Here's how the part is built. I have some questions about the finished solid (model axes, mm). A direction names the side the tool comes from. Give positions to 0.01 mm unless a question says otherwise; leave off trailing zeros. Order: outer loops, then holes, each group sorted by start corner. A loop starts at its lowest first (then second) coordinate and runs counter-clockwise, first axis right, second up. Notation, with made-up numbers: M 34.5,-28 L 45.5,-28 A30 ccw 45.5,3 Z; hole C 22,-2 d5. An arc over 180 degrees is marked long. Use one line per item in the form item = value.
from build123d import *

# Parameters (mm, degrees)
F1_DEPTH  = 14
F2_R      = 3
F3_DEPTH  = 6.001
F4_R      = 1.75
F5_DEPTH  = 10.001
F7_DEPTH  = 6.0010001
F8_R      = 1.75
F9_DEPTH  = 6.001
F11_DEPTH = 10.0010001


with BuildPart() as f1:
    # F0 (on Top) → F1 (new body)
    with BuildSketch(Plane.XY):
        with BuildLine():
            Line((0.5, 11.7459666924), (0.5, 3.9686269666))
            ThreePointArc((0.5, 3.9686269666), (0, -4), (-0.5, 3.9686269666))
            Line((-0.5, 3.9686269666), (-0.5, 11.7459666924))
            Line((-0.5, 11.7459666924), (-2, 11.7459666924))
            Line((-2, 11.7459666924), (-2, 7.7459666924))
            ThreePointArc((-2, 7.7459666924), (-7.9996074848, -0.0792470114), (-1.8461538462, -7.7840680866))
            ThreePointArc((-1.8461538462, -7.7840680866), (0.9223227028, -9.5482422759), (2, -12.6491106407))
            Line((2, -12.6491106407), (2, -16))
            Line((2, -16), (8, -16))
            Line((8, -16), (8, 0))
            ThreePointArc((8, 0), (6.3245553203, 4.8989794856), (2, 7.7459666924))
            Line((2, 7.7459666924), (2, 11.7459666924))
            Line((2, 11.7459666924), (0.5, 11.7459666924))
        make_face()
    extrude(amount=F1_DEPTH)

    # F2 (on face) → F3 (cut, through all)
    with BuildSketch(Plane(origin=(-2, 0, 0), x_dir=(0, -1, 0), z_dir=(-1, 0, 0))):
        with Locations((-7.7459666924, 7)):
            Circle(F2_R)
    extrude(amount=F3_DEPTH, mode=Mode.SUBTRACT)

    # F4 (on face) → F5 (cut, through all)
    with BuildSketch(Plane(origin=(-2, 0, 0), x_dir=(0, -1, 0), z_dir=(-1, 0, 0))):
        with Locations((-7.7459666924, 7)):
            Circle(F4_R)
    extrude(amount=-F5_DEPTH, mode=Mode.SUBTRACT)

    # F6 (on face) → F7 (cut, through all)
    with BuildSketch(Plane.YZ.offset(2)):
        Polygon((3.7459666924, 4.6905989232), (7.7459666924, 2.3811978465), (11.7459666924, 4.6905989232), (11.7459666924, 9.3094010768), (7.7459666924, 11.6188021535), (3.7459666924, 9.3094010768), align=None)
    extrude(amount=F7_DEPTH, mode=Mode.SUBTRACT)

    # F8 (on face) → F9 (cut, through all)
    with BuildSketch(Plane(origin=(2, 0, 0), x_dir=(0, -1, 0), z_dir=(-1, 0, 0))):
        with Locations((12, 7)):
            Circle(F8_R)
    extrude(amount=-F9_DEPTH, mode=Mode.SUBTRACT)

    # F10 (on face) → F11 (cut, through all)
    with BuildSketch(Plane(origin=(2, 0, 0), x_dir=(0, -1, 0), z_dir=(-1, 0, 0))):
        Polygon((15.8407900553, 9.3094010768), (11.8407900553, 11.6188021535), (7.8407900553, 9.3094010768), (7.8407900553, 4.6905989232), (11.8407900553, 2.3811978465), (15.8407900553, 4.6905989232), align=None)
    extrude(amount=F11_DEPTH, mode=Mode.SUBTRACT)


solid = f1.part
Q1. On a 3-axis mill with a long thin cutter (end or side, diameter ignored), from which of +Z, -Z, +X, -X, +Y, -Y can I reach the whole of each face in a straight line? I mean faces 1 (the face through (0.5, 10, 7)), 2 (the face through (2, 9, 5)), 3 (the face through (8, -8, 7)), 4 (the face through (-2, 10, 7)), 5 (the face through (0, -7.841, 7)). Say none if no direction works.
Found:
face_1 = +Z, -Z, +Y
face_2 = +X, +Y
face_3 = +Z, -Z, +X, +Y, -Y
face_4 = -X, +Y
face_5 = -X, -Y
Q2. I want a section at D-D on x = 6.75. Write out the boundary of the cut face in (y, z), then the cut area to 3 significant figures.
Found:
outline = M -16,0 L 4.29,0 L 4.29,4.37 L 3.75,4.69 L 3.75,9.31 L 4.29,9.63 L 4.29,14 L -16,14 Z; hole C -12,7 d3.5
area = 272 mm²
Q3. I want a section at B-B on x = -1.25. Write out the boundary of the cut face in (y, z), then the cut area to 3 significant figures.
Found:
outline = M -7.97,0 L -3.8,0 L -3.8,14 L -7.97,14 L -7.97,9.38 L -7.84,9.31 L -7.84,4.69 L -7.97,4.62 Z; M 3.8,0 L 11.75,0 L 11.75,14 L 3.8,14 Z; hole C 7.75,7 d3.5
area = 159 mm²
Q4. Thinking about a two-plate mould opening in Z: for faces 6 (the face through (-0.5, 10, 7)), 7 (the face through (2, -5, 14)), 8 (the face through (-1.26, 9.135, 5.935)), which applies, +Z half, -Z half, draft (parallel to the pull), parting line (faces both ways), or undercut?
Found:
face_6 = draft
face_7 = +Z half
face_8 = undercut
Q5. I'm going to push flat-ended pins straight in: pin 1 Ø1.8 at (x, z) = (1, 7) entering from -Y; pin 2 Ø5.5 at (y, z) = (-12, 7) entering from -X; pin 3 Ø6.5 at (y, z) = (7.5, 7) entering from +X; pin 4 Ø6.5 at (x, y) = (0, 0) entering from -Z. Where does each tip first touch, or does it pass through?
Found:
pin_1 = -7.84
pin_2 = 2
pin_3 = 2
pin_4 = through
Q6. I want a section at C-C on y = 0.75. Write out the boundary of the cut face in (x, z), then the cut area to 3 significant figures.
Found:
outline = M -7.96,0 L -3.93,0 L -3.93,14 L -7.96,14 Z; M 3.93,0 L 7.96,0 L 7.96,14 L 3.93,14 Z
area = 113 mm²
Q7. I need wall thicknesses on L1, parallel to Y at x = 1, z = 7.75; L2, parallel to Y at x = 4.1, z = 7; L3, parallel to Y at x = -1, z = 7.25. Which ranges of each line are inside material? Lowest first, please.
Found:
L1 = -7.84 to -3.87, 3.87 to 6.16, 9.33 to 11.75
L2 = -16 to -13.75, -10.25 to 3.75
L3 = -7.84 to -3.87, 3.87 to 6.01, 9.48 to 11.75
Q8. I want a section at A-A on z = 7. Write out the boundary of the cut face in (x, y), then the cut area to 3 significant figures.
Found:
outline = M -6.44,4.75 A8 ccw -1.85,-7.78 A5 cw -1.63,-7.84 L 2,-7.84 L 2,-10.25 L 8,-10.25 L 8,0 A8 ccw 7.07,3.75 L 2,3.75 L 2,6 L 0.5,6 L 0.5,3.97 A4 cw long -0.5,3.97 L -0.5,6 L -2,6 L -2,4.75 Z; M -2,9.5 L -0.5,9.5 L -0.5,11.75 L -2,11.75 Z; M 0.5,9.5 L 2,9.5 L 2,11.75 L 0.5,11.75 Z; M 2,-16 L 8,-16 L 8,-13.75 L 2,-13.75 Z
area = 167 mm²
